```python
from build123d import *

# Parameters (mm, degrees)
EXTRUDE_1_DEPTH     = 16
EXTRUDE_2_DEPTH     = 13
SKETCH_4_R          = 6
CUT_EXTRUDE_1_DEPTH = 13
EXTRUDE_3_DEPTH     = 19
CUT_EXTRUDE_2_DEPTH = 35


with BuildPart() as part:
    # 草图1 → 凸台-拉伸1 (new body)
    with BuildSketch(Plane.XY):
        Polygon((0, 0), (-40, 0), (-40, 20), (-14, 52), (0, 52), align=None)
    extrude_1 = extrude(amount=EXTRUDE_1_DEPTH)

    # 镜向1: 凸台-拉伸1 across plane
    add(extrude_1.mirror(Plane(origin=(0, 0, 16), x_dir=(0, 0, 1), z_dir=(-1, 0, 0))))

    # 草图3 → 凸台-拉伸2 (add)
    with BuildSketch(Plane(origin=(0, 52, 0), x_dir=(1, 0, 0), z_dir=(0, 1, 0))):
        with BuildLine():
            Line((-14, 0), (-14, -27))
            ThreePointArc((-14, -27), (0, -41), (14, -27))
            Line((14, -27), (14, 0))
            Line((14, 0), (-14, 0))
        make_face()
    extrude(amount=EXTRUDE_2_DEPTH)

    # 草图4 → 切除-拉伸1 (cut)
    with BuildSketch(Plane(origin=(0, 65, 0), x_dir=(1, 0, 0), z_dir=(0, 1, 0))):
        with Locations(Location((0, -27, 0), (0, 0, 270))):
            Circle(SKETCH_4_R)
    extrude(amount=-CUT_EXTRUDE_1_DEPTH, mode=Mode.SUBTRACT)

    # 草图5 → 凸台-拉伸3 (add)
    with BuildSketch(Plane.XY.offset(16)):
        Polygon((0, 0), (-21, 0), (-21, 12), (-4, 30), (0, 30), align=None)
    extrude_3 = extrude(amount=EXTRUDE_3_DEPTH)

    # 镜向2: 凸台-拉伸3 across plane
    add(extrude_3.mirror(Plane(origin=(0, 0, 35), x_dir=(0, 0, 1), z_dir=(-1, 0, 0))))

    # 草图6 → 切除-拉伸2 (cut)
    with BuildSketch(Plane.XY.offset(35)):
        with BuildLine():
            Line((-12, 0), (12, 0))
            ThreePointArc((12, 0), (0, 12), (-12, 0))
        make_face()
    extrude(amount=-CUT_EXTRUDE_2_DEPTH, mode=Mode.SUBTRACT)


solid = part.part
```
The model under review builds one solid part; all positions refer to its coordinate system, in mm. A direction names the side the tool comes from. Round coordinates to 2 decimals unless told otherwise and drop trailing zeros. Loops run counter-clockwise (first coordinate to the right, second up) from the corner with the lowest first, then second, coordinate; pieces in that order, holes last. Notation, with made-up numbers: M -28,72.25 L 25,72.25 A24 cw 25,88.25 Z; hole C 20,83.25 d8. An arc over 180 degrees is marked long. Put each result on its own line as item: value.
Q1. Consider section D-D, the plane y = 14.5. Give the boundary of the cut face in (x, z).
Result set:
outline: M -40,0 L 40,0 L 40,16 L 18.64,16 L 18.64,35 L -18.64,35 L -18.64,16 L -40,16 Z
Q2. For pin 1 (4 mm diameter, centred on y = 56, z = 9.5, fed in from +X); pin 2 (9.5 mm diameter, centred on y = 9, z = 22.5, fed in from -X); pin 3 (9 mm diameter, centred on x = 1, z = 24, fed in from +Y); pin 4 (1.5 mm diameter, centred on x = 22, z = 10, fed in from +Y), all flat-tipped, find the tip position at first contact; note any pin that passes through.
Result set:
pin 1: stops at x = 14
pin 2: stops at x = -21
pin 3: stops at y = 65
pin 4: stops at y = 43.08
Q3. Mouldability with a two-part tool opening along Y and no side actions: class faces 1 (the flat face through (23, 0, 13)), 2 (the flat face through (27, 36, 8)), 3 (the flat face through (-12.619, 20.874, 25.367)) as released by +Y, released by -Y, zero draft, split by the parting line, or undercut.
Result set:
face 1: released by -Y
face 2: released by +Y
face 3: undercut
Q4. Machinability: for faces 4 (the flat face through (14, 58, 14)), 5 (the flat face through (-1, 32, 16)), 6 (the flat face through (12.619, 20.874, 25.367)), 7 (the flat face through (-21, 6, 25)), which of the approach directions +Z, -Z, +X, -X, +Y, -Y give a long, thin tool a straight path to every point of the face, cutting with its end or side? Answer none if there is none.
Result set:
face 4: +Z, -Z, +X, +Y
face 5: +Z
face 6: +Z, +X
face 7: +Z, -X, +Y, -Y
Q5. Consider section B-B, the plane z = 20. Give the boundary of the cut face in (x, y), then the cut area to 3 significant figures.
Result set:
outline: M -21,0 L -12,0 A12 cw 12,0 L 21,0 L 21,12 L 4,30 L -4,30 L -21,12 Z; M -14,52 L 14,52 L 14,65 L -14,65 Z
area: 1,090 mm²
Q6. To check wall thickness, follow L1, parallel to X at y = 55, z = 27; L2, parallel to X at y = 52.5, z = 31; L3, parallel to Y at x = -1, z = 33. State the ranges of each line that lie inside material, in increasing order.
Result set:
L1: x = -14 to -6, 6 to 14
L2: x = -13.42 to -4.47, 4.47 to 13.42
L3: y = 11.96 to 30, 52 to 65
Q7. Consider section A-A, the plane x = 0. Give the boundary of the cut face in (y, z).
Result set:
outline: M 12,0 L 65,0 L 65,21 L 52,21 L 52,16 L 30,16 L 30,35 L 12,35 Z; M 52,33 L 65,33 L 65,41 L 52,41 Z
Q8. Consider section C-C, the plane y = 55.5. Give the boundary of the cut face in (x, z).
Result set:
outline: M -14,0 L 14,0 L 14,27 A14 ccw -14,27 Z; hole C 0,27 d12
